Geometry: final body of the model. Coordinates: model frame, mm. Face numbers are marked on the shaded views. A direction names the side the tool comes from. Give positions to 0.01 mm unless a question says otherwise; leave off trailing zeros. Order: outer loops, then holes, each group sorted by start corner. A loop starts at its lowest first (then second) coordinate and runs counter-clockwise, first axis right, second up. Notation, with made-up numbers: (15.25, 21.25) -> (42.25, 21.25) arc R26 cw to (42.25, 45.25) -> close; hole circle Ø8 at (-0.5, 2.25). An arc over 180 degrees is marked (long way). Write item = value, one per line.
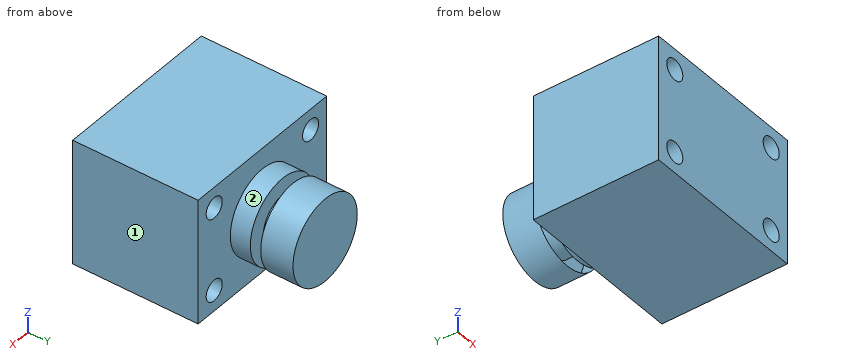
```python
from build123d import *

# Parameters (mm, degrees)
F0_W     = 101.6
F0_H     = 76.2
F1_DEPTH = 76.2
F2_R     = 6.35
F3_DEPTH = 76.201
F4_W     = 25.4
F4_H     = 38.1


with BuildPart() as f1:
    # F0 (on Front) → F1 (new body)
    with BuildSketch(Plane.XZ):
        Rectangle(F0_W, F0_H)
    extrude(amount=F1_DEPTH)

    # F2 (on face) → F3 (cut, through all)
    with BuildSketch(Plane.XZ.offset(76.2)):
        with Locations((-38.1, 25.4)):
            Circle(F2_R)
        with Locations((-38.1, -25.4)):
            Circle(F2_R)
        with Locations((38.1, 25.4)):
            Circle(F2_R)
        with Locations((38.1, -25.4)):
            Circle(F2_R)
    extrude(amount=-F3_DEPTH, mode=Mode.SUBTRACT)

    # F4 (on Top) → F5 (revolve)
    with BuildSketch(Plane.XY):
        with Locations((-12.7, 19.05)):
            Rectangle(F4_W, F4_H)
    revolve(axis=Axis((0, 19.05, 0), (0, -1, 0)))

    # F6 (on Right) → F7 (revolve, cut)
    with BuildSketch(Plane.YZ):
        Polygon((12.171632, -25.511539), (27.484952, -25.241176), (27.484952, -15.148931), (12.171632, -15.148931), align=None)
    revolve(axis=Axis((0, -19.153455, 0), (0, -1, 0)), mode=Mode.SUBTRACT)


solid = f1.part
```
1) Section query D-D (z = 23.5). Count the separate pieces of the cut face and the enclosed holes in it, plus the area to 3 significant figures.
Check sheet entries:
separate_pieces = 4
enclosed_holes = 0
area = 6,340 mm²
2) Section query C-C (y = 17). Output: boundary loops of the cut face in (x, z).
Check sheet entries:
outline = circle Ø30.3 at (0, 0)
3) Reachability of the marked faces 1 and 2 from +Z, -Z, +X, -X, +Y, -Y: full face, straight path, thin tool, end or side. Return the list, or none.
Check sheet entries:
face_1 = +Z, -Z, +X, +Y, -Y
face_2 = +Y
4) Line query: line 1 (Z direction, x = 38.1, y = -22); line 2 (X direction, y = -52, z = 25); line 3 (Z direction, x = -32.5, y = -26). Output: solid intervals per line, ascending. Write a range as from..to.
Check sheet entries:
line_1 = -38.1..-31.75, -19.05..19.05, 31.75..38.1
line_2 = -50.8..-44.44, -31.76..31.76, 44.44..50.8
line_3 = -38.1..-28.39, -22.41..22.41, 28.39..38.1
5) Section query A-A (y = -6). Output: boundary loops of the cut face in (x, z).
Check sheet entries:
outline = (-50.8, -38.1) -> (50.8, -38.1) -> (50.8, 38.1) -> (-50.8, 38.1) -> close; hole circle Ø12.7 at (-38.1, -25.4); hole circle Ø12.7 at (-38.1, 25.4); hole circle Ø12.7 at (38.1, -25.4); hole circle Ø12.7 at (38.1, 25.4)
6) Section query B-B (x = -38.1). Output: boundary loops of the cut face in (y, z), plus the area to 3 significant figures.
Check sheet entries:
outline = (-76.2, -38.1) -> (0, -38.1) -> (0, -31.75) -> (-76.2, -31.75) -> close; (-76.2, -19.05) -> (0, -19.05) -> (0, 19.05) -> (-76.2, 19.05) -> close; (-76.2, 31.75) -> (0, 31.75) -> (0, 38.1) -> (-76.2, 38.1) -> close
area = 3,870 mm²
7) First-contact query: P1, Ø1.5, axis at x = -7.5, y = 3, coming from the -Z side; P2, Ø14.5, axis at x = -38.1, z = 25.4, coming from the -Y side; P3, Ø12, axis at y = 20.5, z = 17.5, coming from the +X side; P4, Ø14.5, axis at x = 38.1, z = 25.4, coming from the +Y side. Flat tips, straight axial feed; report the tip coordinate or a pass-through.
Check sheet entries:
P1 = -24.49
P2 = -76.2
P3 = 22.65
P4 = 0
